Work out the finished part from the listing and answer in its coordinate system (mm). Face numbers are marked on the shaded views. A direction names the side the tool comes from. Coordinates: 2 decimals unless noted, no trailing zeros. Order: outer loops, then holes, each group sorted by start corner. A loop starts at its lowest first (then second) coordinate and runs counter-clockwise, first axis right, second up. Notation, with made-up numbers: (-24.5, 11.5) - (6.5, 11.5) arc R23 ccw to (6.5, 29.5) - close; hole circle Ø4 at (-5, 30.25). An arc over 180 degrees is marked (long way). Answer as a JSON object with one key per item and string values. Group by question number.
1) A tool of negligible diameter and unlimited length cuts with its end or side. For the marked faces 1 and 2, from which of +Z, -Z, +X, -X, +Y, -Y can it reach the whole face along a straight path? Write none if from no direction.
2) Section A-A (y = 5) is taken. Give the vertices of the cut face in (x, z).
3) Section B-B (z = -51) is taken. Give the vertices of the cut face in (x, y).
4) The mould has two halves that part along X. Classify the marked faces 3, 4 and 5: released by +X, released by -X, zero draft, split by the parting line, or undercut.
5) Find the intervals of material crossed by line 1 along X through (y, z) = (17, 32.5); line 2 along Y through (x, z) = (-29, -13.5), in increasing order.
6) Section C-C (x = 26.5) is taken. Give the vertices of the cut face in (y, z), plus the area to 3 significant figures.
7) This flat-tipped pin is pushed along its axis until it touches: P1, Ø2, axis at x = -24, z = 21.5, coming from the +Y side. Where does it stop, or does it pass through?
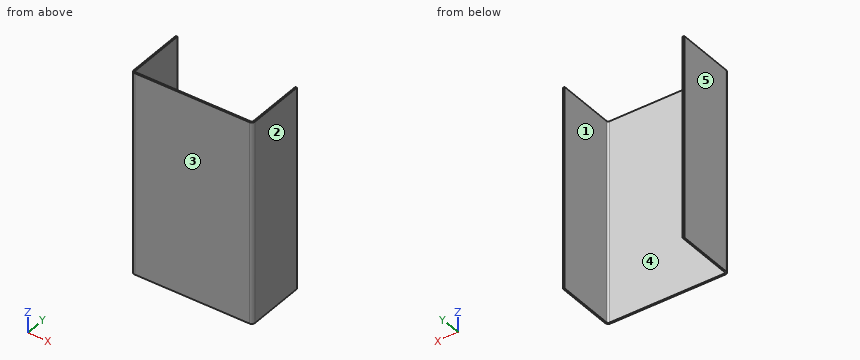
from build123d import *

# Parameters (mm, degrees)
SKETCH_2_W                       = 73.493597356
SKETCH_2_H                       = 125.730953214
SM_BASE_FLANGE_1_DEPTH           = 1
SM_EDGE_FLANGE_1_STRIP_W         = 6
SM_EDGE_FLANGE_1_STRIP_H         = 1
SM_EDGE_FLANGE_1_STRIP_CUT_DEPTH = 125.730953215
SM_EDGE_FLANGE_1_DEPTH           = 125.730953215


# Sheet-metal steps are written as plain solids
with BuildPart() as part:
    # Sketch 2 → Базовая кромка1 (new body)
    with BuildSketch(Plane(origin=(0, 0, 0), x_dir=(1, 0, 0), z_dir=(0, 1, 0))):
        Rectangle(SKETCH_2_W, SKETCH_2_H)
    extrude(amount=-SM_BASE_FLANGE_1_DEPTH)

    # Ребро-кромка1 strip (across the edge) → Ребро-кромка1 strip cut (cut)
    with BuildSketch(Plane(origin=(36.746798678, 0, 62.865476607), x_dir=(-1, 0, 0), z_dir=(0, 0, -1))):
        with Locations((-2, -0.5)):
            Rectangle(SM_EDGE_FLANGE_1_STRIP_W, SM_EDGE_FLANGE_1_STRIP_H)
    sm_edge_flange_1_strip_cut = extrude(amount=SM_EDGE_FLANGE_1_STRIP_CUT_DEPTH, mode=Mode.SUBTRACT)

    # Ребро-кромка1 section (across the edge) → Ребро-кромка1 (add)
    with BuildSketch(Plane(origin=(36.746798678, 0, 62.865476607), x_dir=(-1, 0, 0), z_dir=(0, 0, -1))):
        with BuildLine():
            Line((-1, 1), (-1, 37))
            Line((-1, 37), (0, 37))
            Line((0, 37), (0, 1))
            ThreePointArc((0, 1), (0.292893219, 0.292893219), (1, 0))
            Line((1, 0), (1, -1))
            ThreePointArc((1, -1), (-0.414213562, -0.414213562), (-1, 1))
        make_face()
    sm_edge_flange_1 = extrude(amount=SM_EDGE_FLANGE_1_DEPTH)

    # Зеркальное отражение1: Ребро-кромка1 strip cut, Ребро-кромка1 across plane
    add(sm_edge_flange_1_strip_cut.mirror(Plane(origin=(0, 0, 0), x_dir=(0, 0, 1), z_dir=(1, 0, 0))), mode=Mode.SUBTRACT)
    add(sm_edge_flange_1.mirror(Plane(origin=(0, 0, 0), x_dir=(0, 0, 1), z_dir=(1, 0, 0))))


solid = part.part
Report:
{
 "1": {"face 1": "+Z, -Z, +Y", "face 2": "+Z, -Z, +X, +Y, -Y"},
 "2": {"outline": "(-37.75, -62.87) - (-36.75, -62.87) - (-36.75, 62.87) - (-37.75, 62.87) - close; (36.75, -62.87) - (37.75, -62.87) - (37.75, 62.87) - (36.75, 62.87) - close"},
 "3": {"outline": "(-37.75, 1) arc R2 ccw to (-35.75, -1) - (35.75, -1) arc R2 ccw to (37.75, 1) - (37.75, 37) - (36.75, 37) - (36.75, 1) arc R1 cw to (35.75, 0) - (-35.75, 0) arc R1 cw to (-36.75, 1) - (-36.75, 37) - (-37.75, 37) - close"},
 "4": {"face 3": "zero draft", "face 4": "undercut", "face 5": "released by -X"},
 "5": {"line 1": "x = -37.75 to -36.75, 36.75 to 37.75", "line 2": "y = -1 to 0"},
 "6": {"outline": "(-1, -62.87) - (0, -62.87) - (0, 62.87) - (-1, 62.87) - close", "area": "126 mm²"},
 "7": {"P1": "stops at y = 0"}
}
